```python
from build123d import *

# Parameters (mm, degrees)
M3_CLEARANCE_HOLE1_D = 3.4
FILLET1_R            = 0.2
FILLET2_R            = 0.2
CHAMFER1_SIZE        = 0.5


with BuildPart() as part:
    # Sketch1 → Revolve1 (revolve)
    with BuildSketch(Plane.XY, mode=Mode.PRIVATE) as revolve1_sk:
        Polygon((11, -3), (11, 15.65), (9, 15.65), (9, 18.65), (14, 18.65), (14, 0), (26, 0), (26, -3), align=None)
    revolve(revolve1_sk.sketch.rotate(Axis((0, 17.954019247, 0), (0, -1, 0)), 90), axis=Axis((0, 17.954019247, 0), (0, -1, 0)))

    # Sketch4 → Groove for BS 3673 P4 - B022M, Internal Circlip1 (revolve, cut)
    with BuildSketch(Plane(origin=(0, 17.954019247, 0), x_dir=(0, 0, 1), z_dir=(-1, 0, 0))):
        with BuildLine():
            Line((11.39, -9.404019247), (9.9, -9.404019247))
            Line((9.9, -9.404019247), (9.9, -8.304019247))
            Line((9.9, -8.304019247), (11.39, -8.304019247))
            ThreePointArc((11.39, -8.304019247), (11.467781746, -8.336237501), (11.5, -8.414019247))
            Line((11.5, -8.414019247), (11.5, -9.294019247))
            ThreePointArc((11.5, -9.294019247), (11.467781746, -9.371800993), (11.39, -9.404019247))
        make_face()
    revolve(axis=Axis((0, -32.045980753, 0), (0, 1, 0)), mode=Mode.SUBTRACT)

    # M3 Clearance Hole1 (through all)
    with Locations(Plane(origin=(0, 0, 0), x_dir=(1, 0, 0), z_dir=(0, 1, 0))):
        with Locations((0, 18.5), (18.5, 0), (0, -18.5), (-18.5, 0)):
            Hole(M3_CLEARANCE_HOLE1_D / 2)

    # Fillet1
    fillet1_edges = [part.edges().sort_by_distance(p)[0] for p in [
        (0, 15.65, -11),
    ]]
    fillet(fillet1_edges, radius=FILLET1_R)

    # Fillet2
    fillet2_edges = [part.edges().sort_by_distance(p)[0] for p in [
        (0, 0, -14),
    ]]
    fillet(fillet2_edges, radius=FILLET2_R)

    # Chamfer1
    chamfer1_edges = [part.edges().sort_by_distance(p)[0] for p in [
        (0, 15.65, -9),
        (0, 18.65, -9),
        (0, 18.65, -14),
        (0, 0, -26),
        (0, -3, -26),
        (0, -3, -11),
    ]]
    chamfer(chamfer1_edges, length=CHAMFER1_SIZE)


solid = part.part
```
The model under review builds one solid part; all positions refer to its coordinate system, in mm. A direction names the side the tool comes from. Round coordinates to 2 decimals unless told otherwise and drop trailing zeros. Loops run counter-clockwise (first coordinate to the right, second up) from the corner with the lowest first, then second, coordinate; pieces in that order, holes last. Notation, with made-up numbers: (-29.75, -25.75) -> (7.25, -25.75) arc R14 cw to (7.25, -9.75) -> close; hole circle Ø1 at (64.25, -2). An arc over 180 degrees is marked (long way). Answer as a JSON object with one key per item and string values. Group by question number.
1) For pin 1 Ø3 at (y, z) = (0, -5.5) entering from -X; pin 2 Ø2 at (x, y) = (7.5, 3) entering from +Z; pin 3 Ø2.5 at (x, z) = (18.5, 0) entering from +Y; pin 4 Ø1 at (x, z) = (-20.5, 7.5) entering from +Y, all flat-tipped, find the tip position at first contact; note any pin that passes through.
2) We need section A-A on z = 0. Give the number of separate pieces and of enclosed holes in the cut face, then the cut area to 3 significant figures.
3) We need section B-B on y = 17. Write out the cut boundary in (x, z), then the cut area to 3 significant figures.
4) Mouldability with a two-part tool opening along Y and no side actions: class faces 4 (the face through (10.74, 12.59, -2.38)), 5 (the face through (-9.2, 18.65, 3.2)), 6 (the face through (11.4, 9.1, -1.5)) as released by +Y, released by -Y, zero draft, split by the parting line, or undercut.
5) For line 1 (X direction, y = 8.95, z = 0); line 2 (Y direction, x = -6.5, z = -16.5); line 3 (X direction, y = 3, z = 4.5), list the stretches that pass through material, from the lowest coordinate up. Write a range as [from, to].
6) For faces 1 (the face through (12.4, 9, 6.5)), 2 (the face through (-6.083, 17.164, -6.633)), 3 (the face through (10, 15.65, 0)), list the 3-axis set-ups (+Z, -Z, +X, -X, +Y, -Y) from which the entire face can be reached by the end or side of a thin tool; tool diameter is ignored.
7) We need section C-C on y = 11.5. Write out the cut boundary in (x, z).
Result set:
{
 "1": {"pin 1": "x = -25.68", "pin 2": "z = 12.4", "pin 3": "through", "pin 4": "y = 0"},
 "2": {"separate pieces": "4", "enclosed holes": "0", "area": "191 mm²"},
 "3": {"outline": "circle Ø28 at (0, 0); hole circle Ø18 at (0, 0)", "area": "361 mm²"},
 "4": {"face 4": "zero draft", "face 5": "released by +Y", "face 6": "undercut"},
 "5": {"line 1": "[-14, -11.5], [11.5, 14]", "line 2": "[-3, 0]", "line 3": "[-13.26, -10.04], [10.04, 13.26]"},
 "6": {"face 1": "+Y", "face 2": "+Y, -Y", "face 3": "-Y"},
 "7": {"outline": "circle Ø28 at (0, 0); hole circle Ø22 at (0, 0)"}
}
